Geometry: final body of the model. Coordinates: model frame, mm. Face numbers are marked on the shaded views. A direction names the side the tool comes from. Give positions to 0.01 mm unless a question says otherwise; leave off trailing zeros. Write each loop counter-clockwise with the first axis right and the second up, starting at its lowest first coordinate (ties: lowest second). Pieces come first, ordered by that corner, then holes. Notation, with made-up numbers: M -38.75,30.25 L 17.25,30.25 A14 cw 17.25,47.25 Z; hole C 47,64 d5. An arc over 180 degrees is marked long. Answer as a JSON object with one key per item and string values.
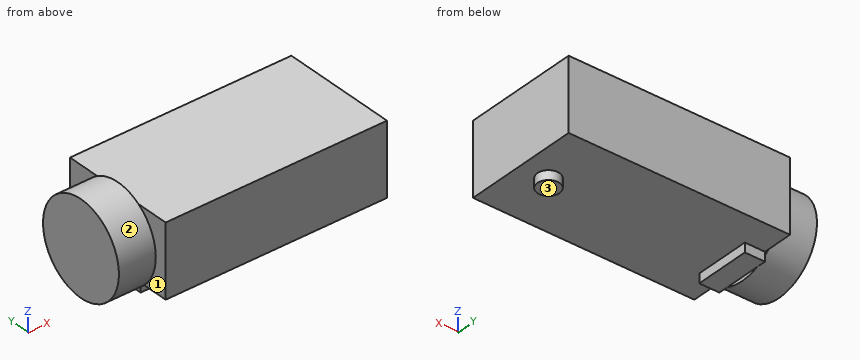
Autodesk Inventor part; units mm, degrees
sketch "スケッチ1" plane through (0, 0, 0) normal (0, 1, 0) x (-1, 0, 0)
  point P0 (0, 0)
sketch "スケッチ2" plane through (0, 0, 0) normal (0, 0, 1) x (1, 0, 0)
  circle A0 centre (10.5, 0) radius 0.6
  line L0 (-2.22, 0) -> (13.32, 0)
  point P0 (0, 0)
  point P1 (0, 0)
  dimension "d0" = 1.2
  dimension "d3" = 10.5
extrude "押し出し1" add sketch "スケッチ2" against normal blind 0.5
sketch "スケッチ4" plane through (0, 0, 0) normal (0, 0, 1) x (1, 0, 0)
  line L0 (12, 3.15) -> (0, 3.15)
  line L1 (0, 3.15) -> (0, -3.15)
  line L2 (0, -3.15) -> (12, -3.15)
  line L3 (12, -3.15) -> (12, 3.15)
  point P0 (0, 0)
  dimension "d4" = 3.15
  dimension "d5" = 6.3
  dimension "d6" = 12
extrude "押し出し2" add sketch "スケッチ4" along normal blind 3.9
sketch "スケッチ5" plane through (0, 0, 0) normal (1, 0, 0) x (0, 1, 0)
  circle A0 centre (0, 1.8) radius 2.5
  point P0 (0, 0)
  dimension "d9" = 5
  dimension "d10" = 1.8
extrude "押し出し3" add sketch "スケッチ5" against normal blind 2
sketch "スケッチ6" plane through (0, 0, 0) normal (0, 0, 1) x (1, 0, 0)
  line L0 (0, -1.5) -> (1.0909, -1.5)
  line L1 (1.0909, -1.5) -> (1.0909, 1.5)
  line L2 (1.0909, 1.5) -> (0, 1.5)
  line L3 (0, 1.5) -> (0, -1.5)
  line L4 (-4.8, 0) -> (14.8, 0)
  point P0 (0, 0)
  dimension "d13" = 3
  dimension "d14" = 1.5
extrude "押し出し4" add sketch "スケッチ6" against normal blind 0.5
properties part number "ST-PJ-312"
1) Line query: line 1 (X direction, y = 2, z = 3.8); line 2 (Z direction, x = 5.5, y = -0.5); line 3 (X direction, y = -1, z = -0.05). Output: solid intervals per line, ascending. Write a range as from..to.
Geometry check:
{"line 1": "x = 0..12", "line 2": "z = 0..3.9", "line 3": "x = -2..1.09"}
2) Cut plane D-D on x = 6.25. Return loops of the section in (y, z).
Geometry check:
{"outline": "M -3.15,0 L 3.15,0 L 3.15,3.9 L -3.15,3.9 Z"}
3) Cut plane B-B on x = 10.5. Return loops of the section in (y, z).
Geometry check:
{"outline": "M -3.15,0 L -0.6,0 L -0.6,-0.5 L 0.6,-0.5 L 0.6,0 L 3.15,0 L 3.15,3.9 L -3.15,3.9 Z"}
4) Set-up query: the marked faces 1, 2 and 3. Return all of +Z, -Z, +X, -X, +Y, -Y with unobstructed straight access to the full face (end or side cutting, diameter ignored); none if empty.
Geometry check:
{"face 1": "-X, -Y", "face 2": "-X", "face 3": "-Z, +X, +Y, -Y"}
5) Cut plane A-A on y = 2. Return loops of the section in (x, z).
Geometry check:
{"outline": "M -2,0.3 L 0,0.3 L 0,0 L 12,0 L 12,3.9 L 0,3.9 L 0,3.3 L -2,3.3 Z"}
6) Contact query for flat-ended pins moving along their axis: P1, Ø1.3, axis at x = 10.5, y = -0.5, coming from the -Z side; P2, Ø2, axis at x = 7, y = -1.5, coming from the +Z side; P3, Ø0.6, axis at x = 0.5, z = -0.5, coming from the +Y side. Output: stop coordinate, or through.
Geometry check:
{"P1": "stops at z = -0.5", "P2": "stops at z = 3.9", "P3": "stops at y = 1.5"}
7) Cut plane C-C on y = 0. Return loops of the section in (x, z), and give its area (3 significant figures).
Geometry check:
{"outline": "M -2,-0.7 L 0,-0.7 L 0,-0.5 L 1.09,-0.5 L 1.09,0 L 9.9,0 L 9.9,-0.5 L 11.1,-0.5 L 11.1,0 L 12,0 L 12,3.9 L 0,3.9 L 0,4.3 L -2,4.3 Z", "area": "57.9 mm2"}
